```python
from build123d import *

# Parameters (mm, degrees)
F1_DEPTH  = 10
F3_DEPTH  = 20
F4_R      = 10
F5_DEPTH  = 93.7
F6_W      = 50
F6_H      = 12
F7_DEPTH  = 6
F10_DEPTH = 28.9


with BuildPart() as f1:
    # F0 (on Top) → F1 (new body)
    with BuildSketch(Plane.XY):
        with BuildLine():
            Line((45.882642, 20), (0, 20))
            ThreePointArc((0, 20), (-20, 0), (0, -20))
            Line((0, -20), (45.882642, -20))
            ThreePointArc((45.882642, -20), (65.882642, 0), (45.882642, 20))
        make_face()
    extrude(amount=F1_DEPTH)

    # F2 (on face) → F3 (join)
    with BuildSketch(Plane.XY.offset(10)):
        with BuildLine():
            ThreePointArc((0, -20), (14.142136, -14.142136), (20, 0))
            ThreePointArc((20, 0), (14.142136, 14.142136), (0, 20))
            ThreePointArc((0, 20), (-20, 0), (0, -20))
        make_face()
    extrude(amount=F3_DEPTH)

    # F4 (on face) → F5 (cut)
    with BuildSketch(Plane.XY.offset(30)):
        Circle(F4_R)
    extrude(amount=-F5_DEPTH, mode=Mode.SUBTRACT)

    # F6 (on face) → F7 (cut)
    with BuildSketch(Plane.XY.offset(30)):
        Rectangle(F6_W, F6_H)
    extrude(amount=-F7_DEPTH, mode=Mode.SUBTRACT)

    # F8 (on face) + F9 (on face) → F10 (cut)
    with BuildSketch(Plane.XY.offset(10)):
        with BuildLine():
            Line((49.295593, 7.5), (34.295593, 7.498614))
            ThreePointArc((34.295593, 7.498614), (26.654353, 0.210243), (33.875122, -7.494909))
            Line((33.875122, -7.494909), (34.422741, -7.49509))
            Line((34.422741, -7.49509), (49.29381, -7.5))
            ThreePointArc((49.29381, -7.5), (56.796286, -0.000891), (49.295593, 7.5))
        make_face()
        with BuildLine():
            Line((34.422741, -7.49509), (33.875122, -7.494909))
            ThreePointArc((33.875122, -7.494909), (34.14893, -7.5), (34.422741, -7.49509))
        make_face()
    with BuildSketch(Plane.XY.offset(10)):
        with BuildLine():
            ThreePointArc((49.29381, -7.5), (56.796286, -0.000891), (49.295593, 7.5))
            Line((49.295593, 7.5), (34.295593, 7.498614))
            ThreePointArc((34.295593, 7.498614), (26.654353, 0.210243), (33.875122, -7.494909))
            Line((33.875122, -7.494909), (34.422741, -7.49509))
            Line((34.422741, -7.49509), (49.29381, -7.5))
        make_face()
    extrude(amount=-F10_DEPTH, mode=Mode.SUBTRACT)


solid = f1.part
```
Geometry check sheet. Reference: the model listing, model coordinates, mm. A direction names the side the tool comes from. Coordinates: 2 decimals unless noted, no trailing zeros. Order: outer loops, then holes, each group sorted by start corner. A loop starts at its lowest first (then second) coordinate and runs counter-clockwise, first axis right, second up.
Q1. Sectioned sample at A-A on z = 4. Record the cut outline in (x, y).
Reply:
outline: (0, -20) - (45.88, -20) arc R20 ccw to (45.88, 20) - (0, 20) arc R20 ccw to start; hole circle Ø20 at (0, 0); hole (33.88, -7.49) arc R7.5 ccw to (34.42, -7.5) - (49.29, -7.5) arc R7.5 ccw to (49.3, 7.5) - (34.3, 7.5) arc R7.5 ccw to start
Q2. Sectioned sample at D-D on z = 11. Record the cut outline in (x, y).
Reply:
outline: (0, -20) arc R20 ccw to (20, 0) arc R20 ccw to (0, 20) arc R20 ccw to start; hole circle Ø20 at (0, 0)
Q3. Sectioned sample at B-B on x = -4. Record the cut outline in (y, z).
Reply:
outline: (-19.6, 0) - (-9.17, 0) - (-9.17, 30) - (-19.6, 30) - close; (9.17, 0) - (19.6, 0) - (19.6, 30) - (9.17, 30) - close
Q4. Thickness scan on probe 1 along X at (y, z) = (0, 8.75); probe 2 along X at (y, z) = (0, 22.25); probe 3 along X at (y, z) = (-3.5, 5.75). Record the ranges inside material, lowest first.
Reply:
probe 1: x = -20 to -10, 10 to 26.65, 56.8 to 65.88
probe 2: x = -20 to -10, 10 to 20
probe 3: x = -19.69 to -9.37, 9.37 to 27.52, 55.93 to 65.57
Q5. Tool access check on faces 5 (the face through (56.794, -0.166, 5.07)), 6 (the face through (23, 20, 5)), 7 (the face through (-14, -6, 27)). Record the directions out of +Z, -Z, +X, -X, +Y, -Y that give a thin tool (end or side, any length) a straight path to the whole face; none if there is none.
Reply:
face 5: +Z, -Z
face 6: +Z, -Z, +X, -X, +Y
face 7: +Z, +X, -X
Q6. Sectioned sample at C-C on y = -2.5. Record the cut outline in (x, z), and give its area (3 significant figures).
Reply:
outline: (-19.84, 0) - (-9.68, 0) - (-9.68, 24) - (-19.84, 24) - close; (9.68, 0) - (27.08, 0) - (27.08, 10) - (19.84, 10) - (19.84, 24) - (9.68, 24) - close; (56.37, 0) - (65.73, 0) - (65.73, 10) - (56.37, 10) - close
area: 654 mm2
Q7. Depth check by flat-ended pin: pin 1 Ø6 at (y, z) = (8, 9.5) entering from +X; pin 2 Ø4 at (x, z) = (23, 12.5) entering from -Y; pin 3 Ø5 at (x, z) = (11.5, 25.5) entering from +Y; pin 4 Ø6.5 at (x, z) = (-12, 27) entering from +Y. Enter the tip coordinate at first touch or a pass-through.
Reply:
pin 1: stops at x = 65.25
pin 2: passes through
pin 3: stops at y = 17.86
pin 4: stops at y = 17.98
Q8. Draft check along Y on faces 1 (the face through (65.878, -0.44, 4.93)), 2 (the face through (13, -6, 27)), 3 (the face through (0, 13, 30)), 4 (the face through (23, -20, 5)). Enter one of: released by +Y, released by -Y, zero draft, split by the parting line, or undercut.
Reply:
face 1: split by the parting line
face 2: undercut
face 3: zero draft
face 4: released by -Y
